Verification items for the finished model (mm, model axes). Coordinates: 2 decimals unless noted, no trailing zeros. Order: outer loops, then holes, each group sorted by start corner. A loop starts at its lowest first (then second) coordinate and runs counter-clockwise, first axis right, second up. Notation, with made-up numbers: M 33.25,13 L 92.25,13 A21 ccw 92.25,38 Z; hole C 45,74.25 d6. An arc over 180 degrees is marked long. Return JSON: item names as keys, results as strings. Group by question number.
1. Section check D-D, the plane y = 3.5. Record the cut outline in (x, z), plus the area to 3 significant figures.
2. Section check C-C, the plane x = -12.7. Record the cut outline in (y, z).
3. Section check B-B, the plane y = -40. Record the cut outline in (x, z), plus the area to 3 significant figures.
4. Gauge pin test, flat end, axial feed: pin 1 (10 mm diameter, centred on x = 38.1, y = 12.7, fed in from -Z). Record the tip position at first contact, or that the pin passes through.
5. Section check A-A, the plane x = -50.8. Record the cut outline in (y, z), plus the area to 3 significant figures.
6. Material ranges on line 1 along Y through (x, z) = (12.7, 0.95); line 2 along Y through (x, z) = (-25, 0.7); line 3 along X through (y, z) = (24, 0.7), recorded low to high.
```python
from build123d import *

# Parameters (mm, degrees)
F0_R     = 6.35
F1_DEPTH = 1.5875


with BuildPart() as f1:
    # F0 (on Top) → F1 (new body)
    with BuildSketch(Plane.XY):
        with BuildLine():
            ThreePointArc((44.45, -50.8), (50.8, -44.45), (57.15, -50.8))
            Line((57.15, -50.8), (63.5, -50.8))
            Line((63.5, -50.8), (63.5, -44.45))
            ThreePointArc((63.5, -44.45), (57.15, -38.1), (63.5, -31.75))
            Line((63.5, -31.75), (63.5, -19.05))
            ThreePointArc((63.5, -19.05), (57.15, -12.7), (63.5, -6.35))
            Line((63.5, -6.35), (63.5, 6.35))
            ThreePointArc((63.5, 6.35), (57.15, 12.7), (63.5, 19.05))
            Line((63.5, 19.05), (63.5, 31.75))
            ThreePointArc((63.5, 31.75), (57.15, 38.1), (63.5, 44.45))
            Line((63.5, 44.45), (63.5, 50.8))
            Line((63.5, 50.8), (57.15, 50.8))
            ThreePointArc((57.15, 50.8), (50.8, 44.45), (44.45, 50.8))
            Line((44.45, 50.8), (31.75, 50.8))
            ThreePointArc((31.75, 50.8), (25.4, 44.45), (19.05, 50.8))
            Line((19.05, 50.8), (6.35, 50.8))
            ThreePointArc((6.35, 50.8), (0, 44.45), (-6.35, 50.8))
            Line((-6.35, 50.8), (-19.05, 50.8))
            ThreePointArc((-19.05, 50.8), (-25.4, 44.45), (-31.75, 50.8))
            Line((-31.75, 50.8), (-44.45, 50.8))
            ThreePointArc((-44.45, 50.8), (-50.8, 44.45), (-57.15, 50.8))
            Line((-57.15, 50.8), (-63.5, 50.8))
            Line((-63.5, 50.8), (-63.5, 44.45))
            ThreePointArc((-63.5, 44.45), (-59.0098719395, 42.5901280605), (-57.15, 38.1))
            ThreePointArc((-57.15, 38.1), (-59.0098719395, 33.6098719395), (-63.5, 31.75))
            Line((-63.5, 31.75), (-63.5, 19.05))
            ThreePointArc((-63.5, 19.05), (-59.0098719395, 17.1901280605), (-57.15, 12.7))
            ThreePointArc((-57.15, 12.7), (-59.0098719395, 8.2098719395), (-63.5, 6.35))
            Line((-63.5, 6.35), (-63.5, -6.35))
            ThreePointArc((-63.5, -6.35), (-59.0098719395, -8.2098719395), (-57.15, -12.7))
            ThreePointArc((-57.15, -12.7), (-59.0098719395, -17.1901280605), (-63.5, -19.05))
            Line((-63.5, -19.05), (-63.5, -31.75))
            ThreePointArc((-63.5, -31.75), (-59.0098719395, -33.6098719395), (-57.15, -38.1))
            ThreePointArc((-57.15, -38.1), (-59.0098719395, -42.5901280605), (-63.5, -44.45))
            Line((-63.5, -44.45), (-63.5, -50.8))
            Line((-63.5, -50.8), (-57.15, -50.8))
            ThreePointArc((-57.15, -50.8), (-50.8, -44.45), (-44.45, -50.8))
            Line((-44.45, -50.8), (-31.75, -50.8))
            ThreePointArc((-31.75, -50.8), (-25.4, -44.45), (-19.05, -50.8))
            Line((-19.05, -50.8), (-6.35, -50.8))
            ThreePointArc((-6.35, -50.8), (0, -44.45), (6.35, -50.8))
            Line((6.35, -50.8), (19.05, -50.8))
            ThreePointArc((19.05, -50.8), (25.4, -44.45), (31.75, -50.8))
            Line((31.75, -50.8), (44.45, -50.8))
        make_face()
        with Locations((-38.1, -38.1)):
            Circle(F0_R, mode=Mode.SUBTRACT)
        with Locations((-12.7, -38.1)):
            Circle(F0_R, mode=Mode.SUBTRACT)
        with Locations((-50.8, -25.4)):
            Circle(F0_R, mode=Mode.SUBTRACT)
        with Locations((-38.1, -12.7)):
            Circle(F0_R, mode=Mode.SUBTRACT)
        with Locations((-25.4, -25.4)):
            Circle(F0_R, mode=Mode.SUBTRACT)
        with Locations((-12.7, -12.7)):
            Circle(F0_R, mode=Mode.SUBTRACT)
        with Locations((12.7, -38.1)):
            Circle(F0_R, mode=Mode.SUBTRACT)
        with Locations((38.1, -38.1)):
            Circle(F0_R, mode=Mode.SUBTRACT)
        with Locations((0, -25.4)):
            Circle(F0_R, mode=Mode.SUBTRACT)
        with Locations((25.4, -25.4)):
            Circle(F0_R, mode=Mode.SUBTRACT)
        with Locations((12.7, -12.7)):
            Circle(F0_R, mode=Mode.SUBTRACT)
        with Locations((50.8, -25.4)):
            Circle(F0_R, mode=Mode.SUBTRACT)
        with Locations((38.1, -12.7)):
            Circle(F0_R, mode=Mode.SUBTRACT)
        with Locations((-50.8, 0)):
            Circle(F0_R, mode=Mode.SUBTRACT)
        with Locations((-38.1, 12.7)):
            Circle(F0_R, mode=Mode.SUBTRACT)
        with Locations((-50.8, 25.4)):
            Circle(F0_R, mode=Mode.SUBTRACT)
        with Locations((-25.4, 0)):
            Circle(F0_R, mode=Mode.SUBTRACT)
        with Locations((-12.7, 12.7)):
            Circle(F0_R, mode=Mode.SUBTRACT)
        with Locations((-25.4, 25.4)):
            Circle(F0_R, mode=Mode.SUBTRACT)
        with Locations((-38.1, 38.1)):
            Circle(F0_R, mode=Mode.SUBTRACT)
        with Locations((-12.7, 38.1)):
            Circle(F0_R, mode=Mode.SUBTRACT)
        Circle(F0_R, mode=Mode.SUBTRACT)
        with Locations((12.7, 12.7)):
            Circle(F0_R, mode=Mode.SUBTRACT)
        with Locations((25.4, 0)):
            Circle(F0_R, mode=Mode.SUBTRACT)
        with Locations((0, 25.4)):
            Circle(F0_R, mode=Mode.SUBTRACT)
        with Locations((25.4, 25.4)):
            Circle(F0_R, mode=Mode.SUBTRACT)
        with Locations((50.8, 0)):
            Circle(F0_R, mode=Mode.SUBTRACT)
        with Locations((38.1, 12.7)):
            Circle(F0_R, mode=Mode.SUBTRACT)
        with Locations((50.8, 25.4)):
            Circle(F0_R, mode=Mode.SUBTRACT)
        with Locations((12.7, 38.1)):
            Circle(F0_R, mode=Mode.SUBTRACT)
        with Locations((38.1, 38.1)):
            Circle(F0_R, mode=Mode.SUBTRACT)
    extrude(amount=F1_DEPTH)


solid = f1.part
```
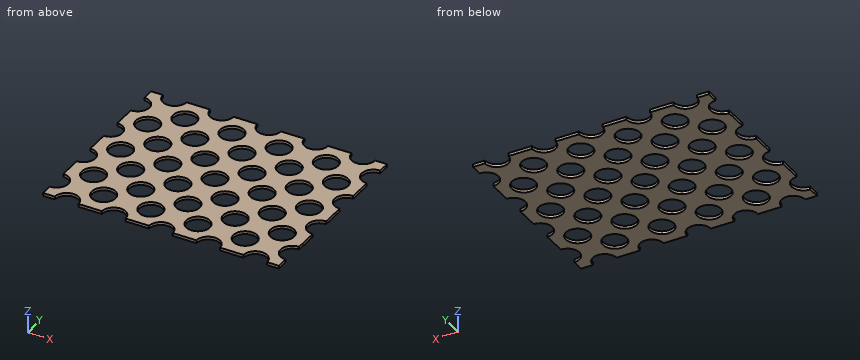
Answers follow:
{
 "1": {"outline": "M -63.5,0 L -56.1,0 L -56.1,1.59 L -63.5,1.59 Z; M -45.5,0 L -30.7,0 L -30.7,1.59 L -45.5,1.59 Z; M -20.1,0 L -5.3,0 L -5.3,1.59 L -20.1,1.59 Z; M 5.3,0 L 20.1,0 L 20.1,1.59 L 5.3,1.59 Z; M 30.7,0 L 45.5,0 L 45.5,1.59 L 30.7,1.59 Z; M 56.1,0 L 63.5,0 L 63.5,1.59 L 56.1,1.59 Z", "area": "118 mm^2"},
 "2": {"outline": "M -50.8,0 L -44.45,0 L -44.45,1.59 L -50.8,1.59 Z; M -31.75,0 L -19.05,0 L -19.05,1.59 L -31.75,1.59 Z; M -6.35,0 L 6.35,0 L 6.35,1.59 L -6.35,1.59 Z; M 19.05,0 L 31.75,0 L 31.75,1.59 L 19.05,1.59 Z; M 44.45,0 L 50.8,0 L 50.8,1.59 L 44.45,1.59 Z"},
 "3": {"outline": "M -57.44,0 L -44.16,0 L -44.16,1.59 L -57.44,1.59 Z; M -32.04,0 L -18.76,0 L -18.76,1.59 L -32.04,1.59 Z; M -6.64,0 L 6.64,0 L 6.64,1.59 L -6.64,1.59 Z; M 18.76,0 L 32.04,0 L 32.04,1.59 L 18.76,1.59 Z; M 44.16,0 L 57.44,0 L 57.44,1.59 L 44.16,1.59 Z", "area": "105 mm^2"},
 "4": {"pin 1": "through"},
 "5": {"outline": "M -44.45,0 L -31.75,0 L -31.75,1.59 L -44.45,1.59 Z; M -19.05,0 L -6.35,0 L -6.35,1.59 L -19.05,1.59 Z; M 6.35,0 L 19.05,0 L 19.05,1.59 L 6.35,1.59 Z; M 31.75,0 L 44.45,0 L 44.45,1.59 L 31.75,1.59 Z", "area": "80.6 mm^2"},
 "6": {"line 1": "-50.8 to -44.45, -31.75 to -19.05, -6.35 to 6.35, 19.05 to 31.75, 44.45 to 50.8", "line 2": "-44.46 to -31.74, -19.06 to -6.34, 6.34 to 19.06, 31.74 to 44.46", "line 3": "-63.5 to -56.99, -44.61 to -31.59, -19.21 to -6.19, 6.19 to 19.21, 31.59 to 44.61, 56.99 to 63.5"}
}
